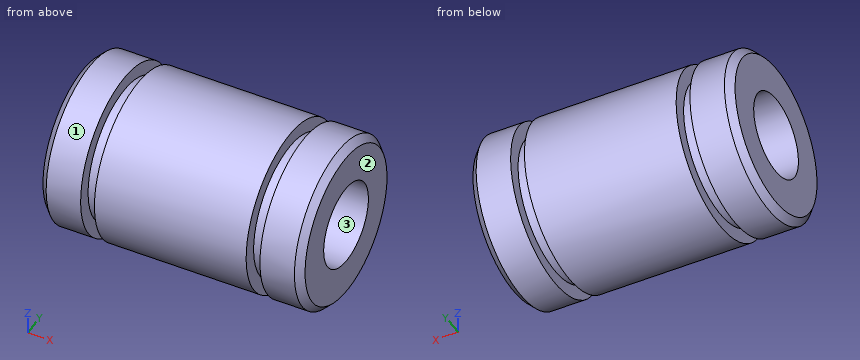
from build123d import *

# Parameters (mm, degrees)
F2_SIZE = 0.5


with BuildPart() as f1:
    # F0 (on Front) → F1 (revolve)
    with BuildSketch(Plane.XZ):
        Polygon((-9.5, 6), (-9.5, 3), (9.5, 3), (9.5, 6), (6.5, 6), (6.5, 5), (5.5, 5), (5.5, 6), (0, 6), (-5.5, 6), (-5.5, 5), (-6.5, 5), (-6.5, 6), align=None)
    revolve(axis=Axis((6.664423, 0, 0), (1, 0, 0)))

    # F2
    f2_edges = [f1.edges().sort_by_distance(p)[0] for p in [
        (-9.5, 0, -6),
        (9.5, 0, -6),
    ]]
    chamfer(f2_edges, length=F2_SIZE)


solid = f1.part
Input: part model. Units: mm. Frame: model coordinates. Face numbers are marked on the shaded views. Give positions to 0.01 mm unless a question says otherwise; leave off trailing zeros. Order: outer loops, then holes, each group sorted by start corner. A loop starts at its lowest first (then second) coordinate and runs counter-clockwise, first axis right, second up. Notation, with made-up numbers: (-19, -32.5) - (22, -32.5) arc R17 cw to (22, -27.5) - close; hole circle Ø9 at (35.5, -17). An arc over 180 degrees is marked (long way). Answer as a JSON object with one key per item and string values. Group by question number.
Q1. Line query: probe 1 along Y at (x, z) = (-4.5, 0); probe 2 along Y at (x, z) = (5.75, 0). Output: solid intervals per line, ascending.
Q2. First-contact query: pin 1 Ø1.5 at (x, z) = (6, 3) entering from -Y; pin 2 Ø1 at (x, y) = (-7, 4.5) entering from -Z; pin 3 Ø3.5 at (y, z) = (0, 0) entering from -X; pin 4 Ø1.5 at (x, z) = (4, 4.5) entering from +Y. Flat tips, straight axial feed; report the tip coordinate or a pass-through.
Q3. Cut plane C-C, the plane x = 4. Output: boundary loops of the cut face in (y, z).
Q4. Cut plane A-A, the plane y = 0. Output: boundary loops of the cut face in (x, z), then the cut area to 4 significant figures.
Q5. Mould query, pull axis Z, two halves, no side actions, for the marked faces 1, 2 and 3. Classes: pulls with the +Z half, pulls with the -Z half, needs draft (parallel to the pull), parting line crosses it, or undercut.
Results:
{
 "1": {"probe 1": "-6 to -3, 3 to 6", "probe 2": "-5 to -3, 3 to 5"},
 "2": {"pin 1": "y = -5.48", "pin 2": "z = -4.47", "pin 3": "through", "pin 4": "y = 4.68"},
 "3": {"outline": "circle Ø12 at (0, 0); hole circle Ø6 at (0, 0)"},
 "4": {"outline": "(-9.5, -5.5) - (-9, -6) - (-6.5, -6) - (-6.5, -5) - (-5.5, -5) - (-5.5, -6) - (5.5, -6) - (5.5, -5) - (6.5, -5) - (6.5, -6) - (9, -6) - (9.5, -5.5) - (9.5, -3) - (-9.5, -3) - close; (-9.5, 3) - (9.5, 3) - (9.5, 5.5) - (9, 6) - (6.5, 6) - (6.5, 5) - (5.5, 5) - (5.5, 6) - (-5.5, 6) - (-5.5, 5) - (-6.5, 5) - (-6.5, 6) - (-9, 6) - (-9.5, 5.5) - close", "area": "109.5 mm^2"},
 "5": {"face 1": "parting line crosses it", "face 2": "needs draft", "face 3": "undercut"}
}
